from build123d import *

# Parameters (mm, degrees)
F0_R     = 120
F0_R_2   = 55
F1_DEPTH = 25
F3_R     = 9
F4_DEPTH = 25
F5_R     = 77.5
F5_R_2   = 55
F6_DEPTH = 5


with BuildPart() as f1:
    # F0 (on Front) → F1 (new body)
    with BuildSketch(Plane.XZ):
        Circle(F0_R)
        Circle(F0_R_2, mode=Mode.SUBTRACT)
    extrude(amount=F1_DEPTH)

    # F3 (on face) → F4 (cut)
    with BuildSketch(Plane.XZ.offset(25)):
        with Locations((0, 100)):
            Circle(F3_R)
        with Locations((-70.710678, 70.710678)):
            Circle(F3_R)
        with Locations((-100, 0)):
            Circle(F3_R)
        with Locations((-70.710678, -70.710678)):
            Circle(F3_R)
        with Locations((0, -100)):
            Circle(F3_R)
        with Locations((70.710678, -70.710678)):
            Circle(F3_R)
        with Locations((100, 0)):
            Circle(F3_R)
        with Locations((70.710678, 70.710678)):
            Circle(F3_R)
    extrude(amount=-F4_DEPTH, mode=Mode.SUBTRACT)

    # F5 (on face) → F6 (join)
    with BuildSketch(Plane.XZ.offset(25)):
        Circle(F5_R)
        Circle(F5_R_2, mode=Mode.SUBTRACT)
    extrude(amount=F6_DEPTH)


solid = f1.part
Here's how the part is built. I have some questions about the finished solid (model axes, mm). A direction names the side the tool comes from. Give positions to 0.01 mm unless a question says otherwise; leave off trailing zeros. Write each loop counter-clockwise with the first axis right and the second up, starting at its lowest first coordinate (ties: lowest second). Pieces come first, ordered by that corner, then holes. Notation, with made-up numbers: (11, 40.5) -> (63, 40.5) arc R23 cw to (63, 54.5) -> close; hole circle Ø5 at (84.5, 59). An arc over 180 degrees is marked (long way). Use one line per item in the form item = value. Start each with the question number.
1. Thinking about a two-plate mould opening in X: for faces 1 (the face through (69.539, -12.675, 79.634)), 2 (the face through (-2, -25, -78)), 3 (the face through (-119.884, -12.325, 5.276)), which applies, +X half, -X half, draft (parallel to the pull), parting line (faces both ways), or undercut?
2. If I drill on L1, parallel to Z at x = 0, y = -19.75; L2, parallel to X at y = -8.25, z = 77.5; L3, parallel to X at y = -24, z = 74.5, over which ranges is the centre line in solid material (lowest first)?
3. Imagine slicing it at A-A on x = 0. List the corners of the cut face in (y, z) for me, plus the area to 4 significant figures.
4. Imagine slicing it at B-B on z = 0. List the corners of the cut face in (x, y) for me.
5. Will these pins go through, and if not, where does the flat tip stop? pin 1 Ø3 at (x, y) = (94.5, -14.5) entering from +Z; pin 2 Ø12 at (y, z) = (-5.5, -64) entering from -X; pin 3 Ø3 at (x, z) = (-67.5, -5) entering from +Y; pin 4 Ø2 at (y, z) = (-8.5, -83) entering from -X.
6. Imagine slicing it at D-D on y = -21. State how many separate pieces and enclosed holes the cut face has, plus the area to 3 significant figures.
7. On a 3-axis mill with a long thin cutter (end or side, diameter ignored), from which of +Z, -Z, +X, -X, +Y, -Y can I reach the whole of each face in a straight line? I mean faces 4 (the face through (-16.8, -27.465, -75.657)), 5 (the face through (75.549, -12.675, -63.122)). Say none if no direction works.
8. Imagine slicing it at C-C on x = -103.5. List the corners of the cut face in (y, z) for me, plus the area to 3 significant figures.
Entries:
q1.face_1 = undercut
q1.face_2 = draft
q1.face_3 = parting line
q2.L1 = -120 to -109, -91 to -55, 55 to 91, 109 to 120
q2.L2 = -91.62 to -76.62, -64.8 to 64.8, 76.62 to 91.62
q2.L3 = -94.07 to -78.87, -62.55 to 62.55, 78.87 to 94.07
q3.outline = (-30, -77.5) -> (-25, -77.5) -> (-25, -91) -> (0, -91) -> (0, -55) -> (-30, -55) -> close; (-30, 55) -> (0, 55) -> (0, 91) -> (-25, 91) -> (-25, 77.5) -> (-30, 77.5) -> close; (-25, -120) -> (0, -120) -> (0, -109) -> (-25, -109) -> close; (-25, 109) -> (0, 109) -> (0, 120) -> (-25, 120) -> close
q3.area = 2,575 mm²
q4.outline = (-120, -25) -> (-109, -25) -> (-109, 0) -> (-120, 0) -> close; (-91, -25) -> (-77.5, -25) -> (-77.5, -30) -> (-55, -30) -> (-55, 0) -> (-91, 0) -> close; (55, -30) -> (77.5, -30) -> (77.5, -25) -> (91, -25) -> (91, 0) -> (55, 0) -> close; (109, -25) -> (120, -25) -> (120, 0) -> (109, 0) -> close
q5.pin_1 = 75.84
q5.pin_2 = -105.05
q5.pin_3 = 0
q5.pin_4 = -87.61
q6.separate_pieces = 1
q6.enclosed_holes = 9
q6.area = 33,700 mm²
q7.face_4 = -Y
q7.face_5 = +Y, -Y
q8.outline = (-25, -60.73) -> (0, -60.73) -> (0, -8.29) -> (-25, -8.29) -> close; (-25, 8.29) -> (0, 8.29) -> (0, 60.73) -> (-25, 60.73) -> close
q8.area = 2,620 mm²
